Can you work these out from the model? Positions are in its coordinate system, mm. A direction names the side the tool comes from. Round coordinates to 2 decimals unless told otherwise and drop trailing zeros. Order: outer loops, then holes, each group sorted by start corner. A loop starts at its lowest first (then second) coordinate and runs counter-clockwise, first axis right, second up. Notation, with made-up numbers: M 82.25,13 L 113.25,13 A36 ccw 113.25,48 Z; hole C 70.25,52.5 d3. An arc over 180 degrees is marked long. Answer as a JSON object with one key per item and string values. Group by question number.
```python
from build123d import *

# Parameters (mm, degrees)
SKETCH1_W                       = 32.2
SKETCH1_H                       = 20.2
BOSS_EXTRUDE1_DEPTH             = 1
BOSS_EXTRUDE2_DEPTH             = 2.5
BOSS_EXTRUDE3_DEPTH             = 2.5
BOSS_EXTRUDE4_REACH             = 18.1
BOSS_EXTRUDE4_DIRECTION_2_REACH = 18.1
BOSS_EXTRUDE5_DEPTH             = 4.5
FILLET1_R                       = 1
SKETCH6_W                       = 1.3
SKETCH6_H                       = 2.4
CUT_EXTRUDE1_DEPTH              = 1


with BuildPart() as part:
    # Sketch1 → Boss-Extrude1 (new body)
    with BuildSketch(Plane(origin=(0, 0, 0), x_dir=(1, 0, 0), z_dir=(0, 1, 0))):
        Rectangle(SKETCH1_W, SKETCH1_H)
    extrude(amount=BOSS_EXTRUDE1_DEPTH)

    # Sketch2 → Boss-Extrude2 (add)
    with BuildSketch(Plane(origin=(0, 1, 0), x_dir=(1, 0, 0), z_dir=(0, 1, 0))):
        Polygon((-16.1, -10.1), (16.1, -10.1), (16.1, -5.5), (15.1, -5.5), (15.1, -9.1), (-15.1, -9.1), (-15.1, 9.1), (15.1, 9.1), (15.1, 5.5), (16.1, 5.5), (16.1, 10.1), (-16.1, 10.1), align=None)
    extrude(amount=BOSS_EXTRUDE2_DEPTH)

    # Sketch3 → Boss-Extrude3 (add)
    with BuildSketch(Plane(origin=(0, 3.5, 0), x_dir=(1, 0, 0), z_dir=(0, 1, 0))):
        Polygon((-10.6, -9.1), (-10.6, -10.1), (16.1, -10.1), (16.1, -5.5), (15.1, -5.5), (15.1, -9.1), align=None)
        Polygon((-16.1, -3.1), (-15.1, -3.1), (-15.1, 9.1), (15.1, 9.1), (15.1, 5.5), (16.1, 5.5), (16.1, 10.1), (-16.1, 10.1), align=None)
    extrude(amount=BOSS_EXTRUDE3_DEPTH)

    # Boss-Extrude4: up to this face of the body (flat: up to its plane)
    boss_extrude4_end = Plane(part.part.faces().sort_by_distance((15.1, 3.5, -7.3))[0])
    # Sketch4 → Boss-Extrude4 (add, up to the picked face)
    with BuildSketch(Plane(origin=(0, 0, 0), x_dir=(0, 0, -1), z_dir=(1, 0, 0)), mode=Mode.PRIVATE) as boss_extrude4_sk1:
        Polygon((-9.1, 6), (-8.8, 5), (-9.1, 4.6), (-9.1, 5), align=None)
    boss_extrude4_tool1 = split(extrude(boss_extrude4_sk1.sketch, amount=BOSS_EXTRUDE4_REACH, mode=Mode.PRIVATE), bisect_by=boss_extrude4_end, keep=Keep.BOTH, mode=Mode.PRIVATE)
    add(boss_extrude4_tool1.solids().sort_by_distance((0, 5.2, 9))[0])
    # Sketch4 → Boss-Extrude4 (add, up to the picked face)
    with BuildSketch(Plane(origin=(0, 0, 0), x_dir=(0, 0, -1), z_dir=(1, 0, 0)), mode=Mode.PRIVATE) as boss_extrude4_sk2:
        Polygon((9.1, 4.6), (9.1, 5), (9.1, 6), (8.8, 5), align=None)
    boss_extrude4_tool2 = split(extrude(boss_extrude4_sk2.sketch, amount=BOSS_EXTRUDE4_REACH, mode=Mode.PRIVATE), bisect_by=boss_extrude4_end, keep=Keep.BOTH, mode=Mode.PRIVATE)
    add(boss_extrude4_tool2.solids().sort_by_distance((0, 5.2, -9))[0])

    # Boss-Extrude4 direction 2: up to this face of the body (flat: up to its plane)
    boss_extrude4_direction_2_end = Plane(part.part.faces().sort_by_distance((-10.6, 4.75, 9.6))[0])
    # Sketch4 → Boss-Extrude4 direction 2 (add, up to the picked face)
    with BuildSketch(Plane(origin=(0, 0, 0), x_dir=(0, 0, -1), z_dir=(1, 0, 0)), mode=Mode.PRIVATE) as boss_extrude4_direction_2_sk1:
        Polygon((-9.1, 6), (-8.8, 5), (-9.1, 4.6), (-9.1, 5), align=None)
    boss_extrude4_direction_2_tool1 = split(extrude(boss_extrude4_direction_2_sk1.sketch, amount=-BOSS_EXTRUDE4_DIRECTION_2_REACH, mode=Mode.PRIVATE), bisect_by=boss_extrude4_direction_2_end, keep=Keep.BOTH, mode=Mode.PRIVATE)
    add(boss_extrude4_direction_2_tool1.solids().sort_by_distance((0, 5.2, 9))[0])
    # Sketch4 → Boss-Extrude4 direction 2 (add, up to the picked face)
    with BuildSketch(Plane(origin=(0, 0, 0), x_dir=(0, 0, -1), z_dir=(1, 0, 0)), mode=Mode.PRIVATE) as boss_extrude4_direction_2_sk2:
        Polygon((9.1, 4.6), (9.1, 5), (9.1, 6), (8.8, 5), align=None)
    boss_extrude4_direction_2_tool2 = split(extrude(boss_extrude4_direction_2_sk2.sketch, amount=-BOSS_EXTRUDE4_DIRECTION_2_REACH, mode=Mode.PRIVATE), bisect_by=boss_extrude4_direction_2_end, keep=Keep.BOTH, mode=Mode.PRIVATE)
    add(boss_extrude4_direction_2_tool2.solids().sort_by_distance((0, 5.2, -9))[0])

    # Sketch5 → Boss-Extrude5 (add)
    with BuildSketch(Plane.ZY.offset(10.6)):
        Polygon((-9.1, 4.6), (-8.8, 5), (-9.1, 6), align=None)
    extrude(amount=BOSS_EXTRUDE5_DEPTH)

    # Fillet1
    fillet1_edges = [part.edges().sort_by_distance(p)[0] for p in [
        (16.1, 3, 10.1),
        (-16.1, 1.75, 10.1),
        (-16.1, 3, -10.1),
        (16.1, 3, -10.1),
    ]]
    fillet(fillet1_edges, radius=FILLET1_R)

    # Sketch6 → Cut-Extrude1 (cut)
    with BuildSketch(Plane.ZY.offset(15.1)):
        with Locations((-8.45, 4.8)):
            Rectangle(SKETCH6_W, SKETCH6_H)
    extrude(amount=CUT_EXTRUDE1_DEPTH, mode=Mode.SUBTRACT)


solid = part.part
```
1) We'd pull the mould along Z, two halves only. Please class faces 4 (the face through (15.6, 3.5, 5.5)), 5 (the face through (-15.6, 4.7, 3.1)), 6 (the face through (-15.4, 3.5, 7.9)): +Z half, -Z half, draft (parallel to the pull), parting line (faces both ways), or undercut.
2) If we section it at A-A on y = 3.95: Write out the boundary of the cut face in (x, z), plus the area to 3 significant figures.
3) If we section it at D-D on x = 5: Write out the boundary of the cut face in (y, z).
4) If we section it at B-B on x = -12.5: Write out the boundary of the cut face in (y, z).
5) I need wall thicknesses on line 1 along X through (y, z) = (2.05, -8.75); line 2 along Z through (x, y) = (5, 1.8); line 3 along Y through (x, z) = (-9, -0.5). Which ranges of each line are inside material? Lowest first, please.
6) If we section it at C-C on z = -6.5: Write out the boundary of the cut face in (x, y).
7) Which directions (+Z, -Z, +X, -X, +Y, -Y) give clear straight access to the entire face, cutting with the end or side of a thin tool? Please do faces 1 (the face through (2.43, 5.507, 8.952)), 2 (the face through (3.7, 6, 9.5)), 3 (the face through (15.6, 3.5, -5.5)).
8) For pin 1 (0.6 mm diameter, centred on y = 5, z = 9.5, fed in from -X); pin 2 (1.7 mm diameter, centred on x = -13.5, z = 7, fed in from +Y); pin 3 (0.8 mm diameter, centred on x = -15.5, y = 4.5, fed in from +Z), each with a flat end and sliding along its axis, tell me the tip position at first contact or that it passes through.
Findings:
{
 "1": {"face 4": "undercut", "face 5": "+Z half", "face 6": "draft"},
 "2": {"outline": "M -16.1,-9.1 A1 ccw -15.1,-10.1 L 15.1,-10.1 A1 ccw 16.1,-9.1 L 16.1,-5.5 L 15.1,-5.5 L 15.1,-9.1 Z; M -16.1,-7.8 L -15.1,-7.8 L -15.1,3.1 L -16.1,3.1 Z; M -10.6,9.1 L 15.1,9.1 L 15.1,5.5 L 16.1,5.5 L 16.1,9.1 A1 ccw 15.1,10.1 L -10.6,10.1 Z", "area": "76.4 mm^2"},
 "3": {"outline": "M 0,-10.1 L 6,-10.1 L 6,-9.1 L 5,-8.8 L 4.6,-9.1 L 1,-9.1 L 1,9.1 L 4.6,9.1 L 5,8.8 L 6,9.1 L 6,10.1 L 0,10.1 Z"},
 "4": {"outline": "M 0,-10.1 L 6,-10.1 L 6,-9.1 L 5,-8.8 L 4.6,-9.1 L 1,-9.1 L 1,9.1 L 3.5,9.1 L 3.5,10.1 L 0,10.1 Z"},
 "5": {"line 1": "x = -16.1 to -15.1, 15.1 to 16.1", "line 2": "z = -10.1 to -9.1, 9.1 to 10.1", "line 3": "y = 0 to 1"},
 "6": {"outline": "M -16.1,0 L 16.1,0 L 16.1,6 L 15.1,6 L 15.1,1 L -15.1,1 L -15.1,6 L -16.1,6 Z"},
 "7": {"face 1": "-X, +Y", "face 2": "+Z, -Z, +X, -X, +Y", "face 3": "+X, +Y"},
 "8": {"pin 1": "stops at x = -10.6", "pin 2": "stops at y = 1", "pin 3": "stops at z = 3.1"}
}
